Can you work these out from the model? Positions are in its coordinate system, mm. Coordinates: 2 decimals unless noted, no trailing zeros. Order: outer loops, then holes, each group sorted by start corner. A loop starts at its lowest first (then second) coordinate and runs counter-clockwise, first axis right, second up. Notation, with made-up numbers: (20.5, -12) -> (29.5, -12) arc R28 cw to (29.5, 16) -> close; hole circle Ø4 at (46.5, 14.5). An arc over 180 degrees is marked (long way). Return JSON: item names as keys, results as strings. Group by question number.
1) If we section it at C-C, the plane y = -3.75: Please give me the cut outline in (x, z), then the cut area to 3 significant figures.
2) If we section it at A-A, the plane z = -29: Please give me the cut outline in (x, y).
3) If we section it at B-B, the plane x = -23: Please give me the cut outline in (y, z), then the cut area to 3 significant figures.
4) If I drill on probe 1 along X at (y, z) = (-4.25, -23); probe 2 along X at (y, z) = (-1.25, -48); probe 3 along X at (y, z) = (-7, -47.5), over which ranges is the centre line in solid material (lowest first)? Write a range as from..to.
from build123d import *

# Parameters (mm, degrees)
F0_W     = 110
F0_H     = 38
F1_DEPTH = 8
F2_W     = 50
F2_H     = 15
F3_DEPTH = 25
F4_D     = 4.4


with BuildPart() as f1:
    # F0 (on Front) → F1 (new body)
    with BuildSketch(Plane.XZ):
        with Locations((-0.1309809089, -36.948600173)):
            Rectangle(F0_W, F0_H)
    extrude(amount=F1_DEPTH)

    # F2 (on face) → F3 (cut)
    with BuildSketch(Plane.XZ.offset(8)):
        with Locations((-0.0620441511, -25.448600173)):
            Rectangle(F2_W, F2_H)
    extrude(amount=-F3_DEPTH, mode=Mode.SUBTRACT)

    # F4 (through all)
    with Locations(Plane(origin=(0, 0, 0), x_dir=(1, 0, 0), z_dir=(0, 1, 0))):
        with Locations((-23, 48.948600173), (23, 48.948600173)):
            Hole(F4_D / 2)

    # F5: F1 across plane


with BuildPart() as f1_1:
    add(f1.part)
    add(f1.part.mirror(Plane.YZ))


solid = f1_1.part
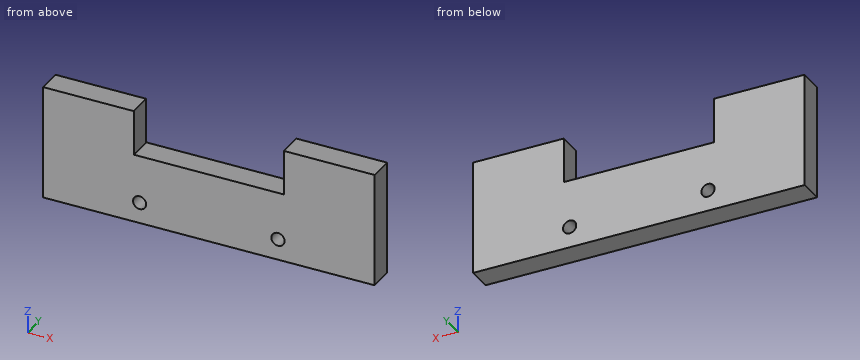
Result sheet:
{
 "1": {"outline": "(-55.13, -55.95) -> (55.13, -55.95) -> (55.13, -17.95) -> (24.94, -17.95) -> (24.94, -32.95) -> (-24.94, -32.95) -> (-24.94, -17.95) -> (-55.13, -17.95) -> close; hole circle Ø4.4 at (-23, -48.95); hole circle Ø4.4 at (23, -48.95)", "area": "3,410 mm2"},
 "2": {"outline": "(-55.13, -8) -> (-24.94, -8) -> (-24.94, 0) -> (-55.13, 0) -> close; (24.94, -8) -> (55.13, -8) -> (55.13, 0) -> (24.94, 0) -> close"},
 "3": {"outline": "(-8, -55.95) -> (0, -55.95) -> (0, -51.15) -> (-8, -51.15) -> close; (-8, -46.75) -> (0, -46.75) -> (0, -32.95) -> (-8, -32.95) -> close", "area": "149 mm2"},
 "4": {"probe 1": "x = -55.13..-24.94, 24.94..55.13", "probe 2": "x = -55.13..-24.98, -21.02..21.02, 24.98..55.13", "probe 3": "x = -55.13..-24.66, -21.34..21.34, 24.66..55.13"}
}
